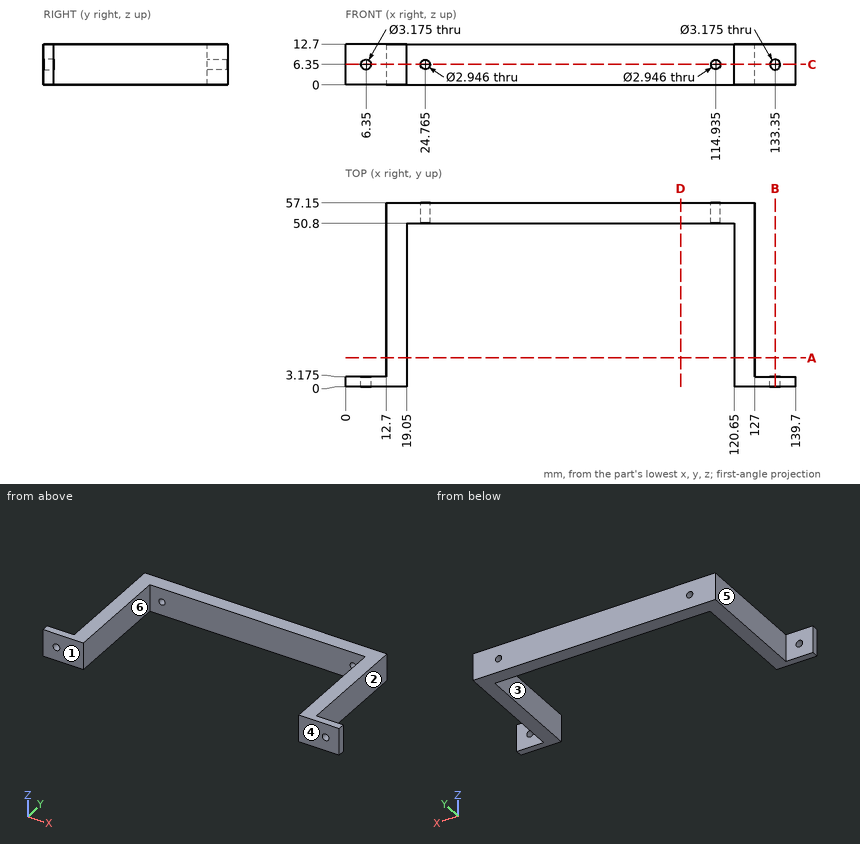
Here's the drawing with two shaded views (mm, measured from the low corner). I have some questions. A direction names the side the tool comes from. Coordinates: 2 decimals unless noted, no trailing zeros. Order: outer loops, then holes, each group sorted by start corner. A loop starts at its lowest first (then second) coordinate and runs counter-clockwise, first axis right, second up.
Q1. Suppose I cut it at A-A on y = 9. Please give me the cut outline in (x, z), and give its area (3 significant figures).
Q2. Suppose I cut it at D-D on x = 104. Please give me the cut outline in (y, z).
Q3. Suppose I cut it at B-B on x = 133.35. Please give me the cut outline in (y, z) (1 decimal).
Q4. Thinking about a two-plate mould opening in X: for the marked faces 1, 2 and 3, which applies, released by +X, released by -X, zero draft, split by the parting line, or undercut?
Q5. Please list where these lines run through material, in increasing order: L1, parallel to X at y = 1.2, z = 6.35; L2, parallel to X at y = 38, z = 7; L3, parallel to Z at x = 6.35, y = 0.6.
Q6. Will these pins go through, and if not, where does the flat tip stop? pin 1 (6.5 mm diameter, centred on y = 32, z = 4, fed in from -X); pin 2 (2 mm diameter, centred on x = 49, z = 3, fed in from -Y); pin 3 (1 mm diameter, centred on y = 31.5, z = 4.5, fed in from +X); pin 4 (4.5 mm diameter, centred on x = 114.935, z = 6.35, fed in from +Y).
Q7. Which directions (+Z, -Z, +X, -X, +Y, -Y) give clear straight access to the entire face, cutting with the end or side of a thin tool? Please do the marked faces 4, 5 and 6.
Q8. Suppose I cut it at C-C on z = 6.35. Give the number of separate pieces and of enclosed holes in the cut face, and give its area (3 significant figures).
Answer:
1. outline: (12.7, 0) - (19.05, 0) - (19.05, 12.7) - (12.7, 12.7) - close; (120.65, 0) - (127, 0) - (127, 12.7) - (120.65, 12.7) - close
1. area: 161 mm2
2. outline: (50.8, 0) - (57.15, 0) - (57.15, 12.7) - (50.8, 12.7) - close
3. outline: (0, 0) - (3.2, 0) - (3.2, 4.8) - (0, 4.8) - close; (0, 7.9) - (3.2, 7.9) - (3.2, 12.7) - (0, 12.7) - close
4. face 1: zero draft
4. face 2: released by +X
4. face 3: undercut
5. L1: x = 0 to 4.76, 7.94 to 19.05, 120.65 to 131.76, 134.94 to 139.7
5. L2: x = 12.7 to 19.05, 120.65 to 127
5. L3: z = 0 to 4.76, 7.94 to 12.7
6. pin 1: stops at x = 12.7
6. pin 2: stops at y = 50.8
6. pin 3: stops at x = 127
6. pin 4: stops at y = 57.15
7. face 4: +Z, -Z, +X, -X, -Y
7. face 5: +Z, -Z, -X, +Y
7. face 6: +Z, -Z, -Y
8. separate pieces: 5
8. enclosed holes: 0
8. area: 1,390 mm2
